Source: three-view drawing plus pictorial views. Frame: mm from the lowest corner of the part. Give positions to 0.01 mm unless a question says otherwise; leave off trailing zeros. Loops run counter-clockwise (first coordinate to the right, second up) from the corner with the lowest first, then second, coordinate; pieces in that order, holes last. Notation, with made-up numbers: (35.5, 41.25) - (50.5, 41.25) arc R19 cw to (50.5, 60.25) - close; hole circle Ø4 at (15.25, 72). An arc over 180 degrees is marked (long way). Put each result on its own line as item: value.
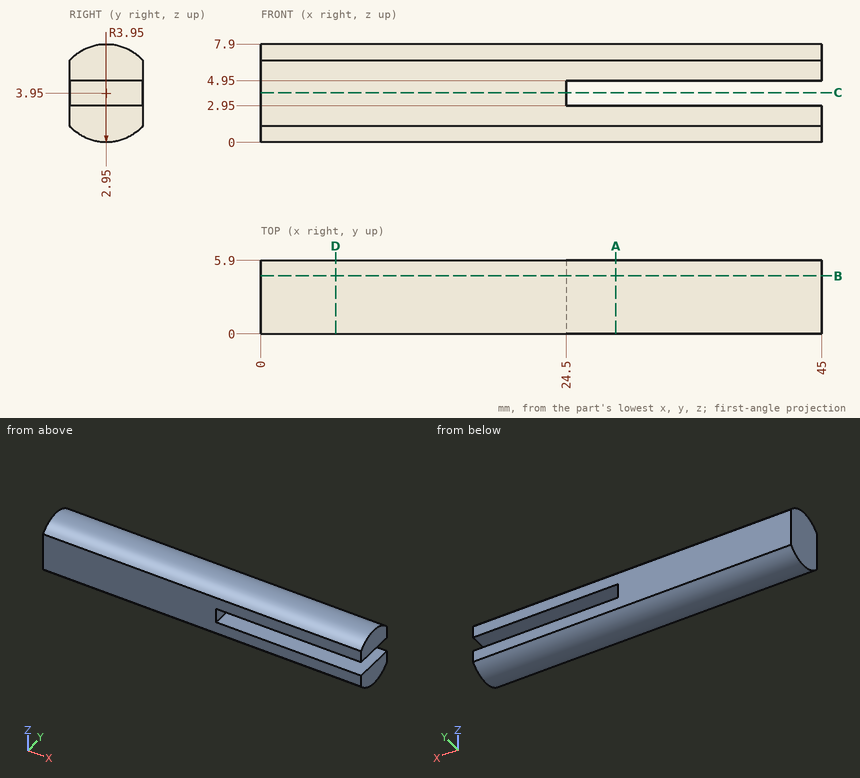
1) Section query B-B, the plane y = 4.65. Output: boundary loops of the cut face in (x, z), plus the area to 3 significant figures.
Check result:
outline: (0, 0.38) - (45, 0.38) - (45, 2.95) - (24.5, 2.95) - (24.5, 4.95) - (45, 4.95) - (45, 7.52) - (0, 7.52) - close
area: 280 mm²
2) Section query D-D, the plane x = 6. Output: boundary loops of the cut face in (y, z).
Check result:
outline: (0, 1.32) arc R3.95 ccw to (5.9, 1.32) - (5.9, 6.58) arc R3.95 ccw to (0, 6.58) - close
3) Section query A-A, the plane x = 28.5. Output: boundary loops of the cut face in (y, z).
Check result:
outline: (0, 1.32) arc R3.95 ccw to (5.9, 1.32) - (5.9, 2.95) - (0, 2.95) - close; (0, 4.95) - (5.9, 4.95) - (5.9, 6.58) arc R3.95 ccw to (0, 6.58) - close
4) Pin query (flat end, axial travel): P1, Ø3, axis at y = 5, z = 3, coming from the +X side; P2, Ø1.8, axis at x = 29.5, y = 4.5, coming from the +Z side. Return the tip coordinate at first contact, or that it passes through.
Check result:
P1: x = 45
P2: z = 7.85
5) Material intervals for line 1 along Z through (x, y) = (11, 3.1); line 2 along Z through (x, y) = (38, 3.85); line 3 along X through (y, z) = (0.65, 3), sorted ascending. Write a range as [from, to].
Check result:
line 1: [0, 7.9]
line 2: [0.1, 2.95], [4.95, 7.8]
line 3: [0, 24.5]
6) Section query C-C, the plane z = 4. Output: boundary loops of the cut face in (x, y), plus the area to 3 significant figures.
Check result:
outline: (0, 0) - (24.5, 0) - (24.5, 5.9) - (0, 5.9) - close
area: 145 mm²
